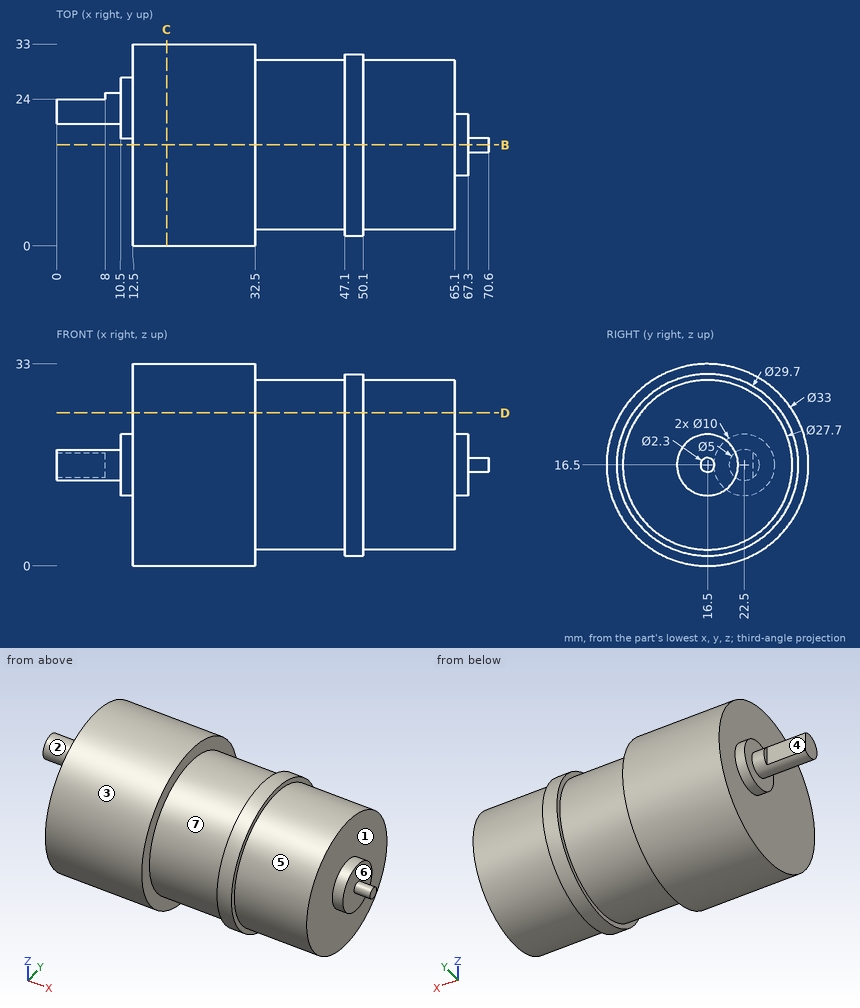
Design review of the part shown in the three views and the two pictorial views. Dimensions are in mm from the part's minimum x, y and z. A direction names the side the tool comes from. Coordinates: 2 decimals unless noted, no trailing zeros. Write each loop counter-clockwise with the first axis right and the second up, starting at its lowest first coordinate (ties: lowest second). Pieces come first, ordered by that corner, then holes.
1) We need section D-D on z = 25. State the section outline as (x, y) points, then the cut area to 3 significant figures.
2) We need section C-C on x = 18. State the section outline as (y, z) points.
3) We need section B-B on y = 16.5. State the section outline as (x, z) points, then the cut area to 3 significant figures.
4) The part is to be moulded in two halves that separate along X. For the marked faces 5, 6 and 7, say which applies: pulls with the +X half, pulls with the -X half, needs draft (parallel to the pull), parting line crosses it, or undercut.
5) Machinability: for the marked faces 1, 2, 3 and 4, which of the approach directions +Z, -Z, +X, -X, +Y, -Y give a long, thin tool a straight path to every point of the face, cutting with its end or side? Answer none if there is none.
6) Clearance check with flat-ended pins moving along their axes: pin 1 Ø3 at (x, z) = (50, 11.5) entering from +Y; pin 2 Ø1.5 at (x, z) = (60, 8.5) entering from +Y; pin 3 Ø8 at (y, z) = (23, 15.5) entering from -X; pin 4 Ø5 at (x, y) = (63, 21) entering from -Z. State where each tip first meets the part, or that it passes through.
7) To check wall thickness, follow probe 1 along X at (y, z) = (28, 7.5); probe 2 along X at (y, z) = (26, 28); probe 3 along X at (y, z) = (5.5, 17). State the ranges of each line that lie inside material, in increasing order.
Answer list:
1. outline: (12.5, 2.36) - (32.5, 2.36) - (32.5, 5.57) - (47.1, 5.57) - (47.1, 4.32) - (50.1, 4.32) - (50.1, 5.57) - (65.1, 5.57) - (65.1, 27.43) - (50.1, 27.43) - (50.1, 28.68) - (47.1, 28.68) - (47.1, 27.43) - (32.5, 27.43) - (32.5, 30.64) - (12.5, 30.64) - close
1. area: 1,290 mm2
2. outline: circle Ø33 at (16.5, 16.5)
3. outline: (12.5, 0) - (32.5, 0) - (32.5, 2.65) - (47.1, 2.65) - (47.1, 1.65) - (50.1, 1.65) - (50.1, 2.65) - (65.1, 2.65) - (65.1, 11.5) - (67.3, 11.5) - (67.3, 15.35) - (70.6, 15.35) - (70.6, 17.65) - (67.3, 17.65) - (67.3, 21.5) - (65.1, 21.5) - (65.1, 30.35) - (50.1, 30.35) - (50.1, 31.35) - (47.1, 31.35) - (47.1, 30.35) - (32.5, 30.35) - (32.5, 33) - (12.5, 33) - close
3. area: 1,600 mm2
4. face 5: needs draft
4. face 6: pulls with the +X half
4. face 7: undercut
5. face 1: +X
5. face 2: -X
5. face 3: +X, -X
5. face 4: +Z, -Z, -X, +Y
6. pin 1: stops at y = 30.93
6. pin 2: stops at y = 28.3
6. pin 3: stops at x = 0
6. pin 4: stops at z = 2.8
7. probe 1: x = 12.5 to 32.5, 47.1 to 50.1
7. probe 2: x = 12.5 to 32.5
7. probe 3: x = 12.5 to 65.1
